Verification items for the finished model (mm, model axes). Coordinates: 2 decimals unless noted, no trailing zeros. Loops run counter-clockwise (first coordinate to the right, second up) from the corner with the lowest first, then second, coordinate; pieces in that order, holes last. Notation, with made-up numbers: (50.25, 85) - (74.25, 85) arc R25 ccw to (74.25, 112) - close; hole circle Ø3 at (-1, 13.5). An arc over 180 degrees is marked (long way). One line per item, written item: value. Start each with the question number.
(1) Section check A-A (y = -11.5). Record the boundary of the cut face in (x, z), plus the area to 3 significant figures.
(2) Section check B-B (x = -54). Record the boundary of the cut face in (y, z), plus the area to 3 significant figures.
(3) Gauge pin test, flat end, axial feed: P1, Ø5, axis at x = -32, y = -11.5, coming from the -Z side. Record the tip position at first contact, or that the pin passes through.
(4) Thickness scan on probe 1 along X at (y, z) = (-19, 17); probe 2 along Z at (x, y) = (-44.5, -9.5); probe 3 along X at (y, z) = (6.5, 34). Record the ranges inside material, lowest first. Write a range as [from, to].
(5) Section check C-C (z = 26). Record the boundary of the cut face in (x, y).
```python
from build123d import *

# Parameters (mm, degrees)
F1_DEPTH = 29


with BuildPart() as f1:
    # F0 (on Front) → F1 (new body, symmetric)
    with BuildSketch(Plane.XZ):
        with BuildLine():
            Line((-63.5, 0), (63.5, 0))
            Line((63.5, 0), (63.5, 9))
            ThreePointArc((63.5, 9), (55.006097, 29.506097), (34.5, 38))
            Line((34.5, 38), (-34.5, 38))
            ThreePointArc((-34.5, 38), (-55.006097, 29.506097), (-63.5, 9))
            Line((-63.5, 9), (-63.5, 0))
        make_face()
    extrude(amount=F1_DEPTH, both=True)


solid = f1.part
```
Responses:
1. outline: (-63.5, 0) - (63.5, 0) - (63.5, 9) arc R29 ccw to (34.5, 38) - (-34.5, 38) arc R29 ccw to (-63.5, 9) - close
1. area: 4,470 mm²
2. outline: (-29, 0) - (29, 0) - (29, 30.47) - (-29, 30.47) - close
2. area: 1,770 mm²
3. P1: stops at z = 0
4. probe 1: x = [-62.37, 62.37]
4. probe 2: z = [0, 36.22]
4. probe 3: x = [-49.2, 49.2]
5. outline: (-57.99, -29) - (57.99, -29) - (57.99, 29) - (-57.99, 29) - close
